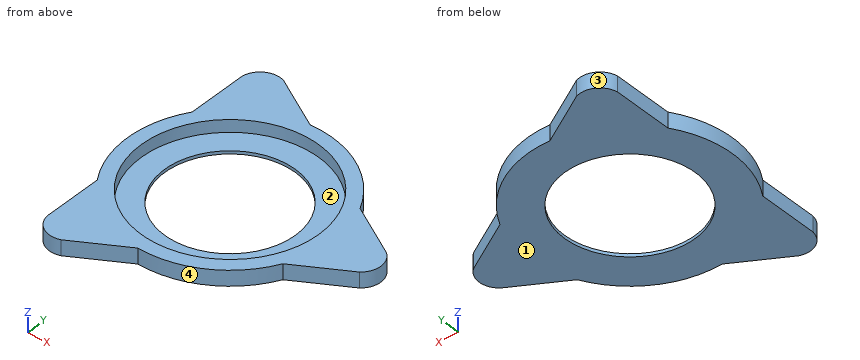
from build123d import *

# Parameters (mm, degrees)
SKETCH1_R          = 40.456394747
BASE_EXTRUDE_DEPTH = 9.525
SKETCH2_R          = 54.991944722
CUT_EXTRUDE1_DEPTH = 7.62


with BuildPart() as part:
    # Sketch1 → Base-Extrude (new body)
    with BuildSketch(Plane.XY):
        with BuildLine():
            Line((88.84522521, -9.917986872), (56.779605871, -28.43108083))
            ThreePointArc((56.779605871, -28.43108083), (31.75, -54.99261314), (-3.76776468, -63.388121516))
            Line((-3.76776468, -63.388121516), (-35.833384019, -81.901215473))
            ThreePointArc((-35.833384019, -81.901215473), (-46.806394747, -81.07105382), (-53.011841191, -71.983228601))
            Line((-53.011841191, -71.983228601), (-53.011841191, -34.957040686))
            ThreePointArc((-53.011841191, -34.957040686), (-63.5, 0), (-53.011841191, 34.957040686))
            Line((-53.011841191, 34.957040686), (-53.011841191, 71.983228601))
            ThreePointArc((-53.011841191, 71.983228601), (-46.806394747, 81.07105382), (-35.833384019, 81.901215473))
            Line((-35.833384019, 81.901215473), (-3.76776468, 63.388121516))
            ThreePointArc((-3.76776468, 63.388121516), (31.75, 54.99261314), (56.779605871, 28.43108083))
            Line((56.779605871, 28.43108083), (88.84522521, 9.917986872))
            ThreePointArc((88.84522521, 9.917986872), (93.612789493, 0), (88.84522521, -9.917986872))
        make_face()
        Circle(SKETCH1_R, mode=Mode.SUBTRACT)
    extrude(amount=BASE_EXTRUDE_DEPTH)

    # Sketch2 → Cut-Extrude1 (cut)
    with BuildSketch(Plane.XY.offset(9.525)):
        Circle(SKETCH2_R)
    extrude(amount=-CUT_EXTRUDE1_DEPTH, mode=Mode.SUBTRACT)


solid = part.part
For this review, take the finished solid that the model builds, in its own axes (mm). Face numbers are marked on the shaded views. Round coordinates to 2 decimals unless told otherwise and drop trailing zeros. Write each loop counter-clockwise with the first axis right and the second up, starting at its lowest first coordinate (ties: lowest second). Pieces come first, ordered by that corner, then holes. Notation, with made-up numbers: (-34, -0.5) - (-27, -0.5) arc R23 cw to (-27, 8.5) - close; hole circle Ø2 at (63.25, 84). An arc over 180 degrees is marked (long way). Use a Markdown table: item, result.
Q1. We need section D-D (y = 42.5). Give the boundary of the cut face in (x, z) (1 decimal).
Derived:
| item | result |
|---|---|
| outline | (-53, 0) - (47.2, 0) - (47.2, 9.5) - (34.9, 9.5) - (34.9, 1.9) - (-34.9, 1.9) - (-34.9, 9.5) - (-53, 9.5) - close |
Q2. Clearance check with flat-ended pins moving along their axes: pin 1 (2 mm diameter, centred on y = 58.5, z = 3.5, fed in from +X); pin 2 (4 mm diameter, centred on x = -13.5, z = 2.5, fed in from -Y); pin 3 (1.5 mm diameter, centred on x = -42.5, y = 30, fed in from +Z) (3 decimals). State where each tip first meets the part, or that it passes through.
Derived:
| item | result |
|---|---|
| pin 1 | stops at x = 26.94 |
| pin 2 | stops at y = -70.16 |
| pin 3 | stops at z = 1.905 |
Q3. Wall thickness on line 1 along X through (y, z) = (0, 0.8); line 2 along Y through (x, z) = (0, 1.4); line 3 along Y through (x, z) = (0, 6.5): over which ranges is each line inside the solid? List them lowest first.
Derived:
| item | result |
|---|---|
| line 1 | x = -63.5 to -40.46, 40.46 to 93.61 |
| line 2 | y = -63.5 to -40.46, 40.46 to 63.5 |
| line 3 | y = -63.5 to -54.99, 54.99 to 63.5 |
Q4. We need section C-C (z = 7.5). Give the boundary of the cut face in (x, y), plus the area to 3 significant figures.
Derived:
| item | result |
|---|---|
| outline | (-53.01, -71.98) arc R12.7 ccw to (-35.83, -81.9) - (-3.77, -63.39) arc R63.5 ccw to (56.78, -28.43) - (88.85, -9.92) arc R12.7 ccw to (88.85, 9.92) - (56.78, 28.43) arc R63.5 ccw to (-3.77, 63.39) - (-35.83, 81.9) arc R12.7 ccw to (-53.01, 71.98) - (-53.01, 34.96) arc R63.5 ccw to (-53.01, -34.96) - close; hole circle Ø109.98 at (0, 0) |
| area | 6,280 mm2 |
Q5. The part is to be moulded in two halves that separate along Y. For the marked faces 1, 2, 3 and 4, say which applies: pulls with the +Y half, pulls with the -Y half, needs draft (parallel to the pull), parting line crosses it, or undercut.
Derived:
| item | result |
|---|---|
| face 1 | needs draft |
| face 2 | undercut |
| face 3 | pulls with the +Y half |
| face 4 | pulls with the -Y half |
Q6. We need section B-B (x = 0). Give the boundary of the cut face in (y, z) (3 decimals).
Derived:
| item | result |
|---|---|
| outline | (-63.5, 0) - (-40.456, 0) - (-40.456, 1.905) - (-54.992, 1.905) - (-54.992, 9.525) - (-63.5, 9.525) - close; (40.456, 0) - (63.5, 0) - (63.5, 9.525) - (54.992, 9.525) - (54.992, 1.905) - (40.456, 1.905) - close |
Q7. We need section A-A (y = 0). Give the boundary of the cut face in (x, z) (3 decimals).
Derived:
| item | result |
|---|---|
| outline | (-63.5, 0) - (-40.456, 0) - (-40.456, 1.905) - (-54.992, 1.905) - (-54.992, 9.525) - (-63.5, 9.525) - close; (40.456, 0) - (93.613, 0) - (93.613, 9.525) - (54.992, 9.525) - (54.992, 1.905) - (40.456, 1.905) - close |
